Print and shaded views of the part. All mm, measured from the part's lowest x, y and z. A direction names the side the tool comes from. Give positions to 0.01 mm unless a question says otherwise; leave off trailing zeros. Order: outer loops, then holes, each group sorted by start corner. A loop starts at its lowest first (then second) coordinate and runs counter-clockwise, first axis right, second up. Notation, with made-up numbers: (36, 73) - (85, 73) arc R20 ccw to (85, 95) - close; hole circle Ø11 at (48, -12.75). An arc over 180 degrees is marked (long way). Answer in a Markdown table with one row per item.
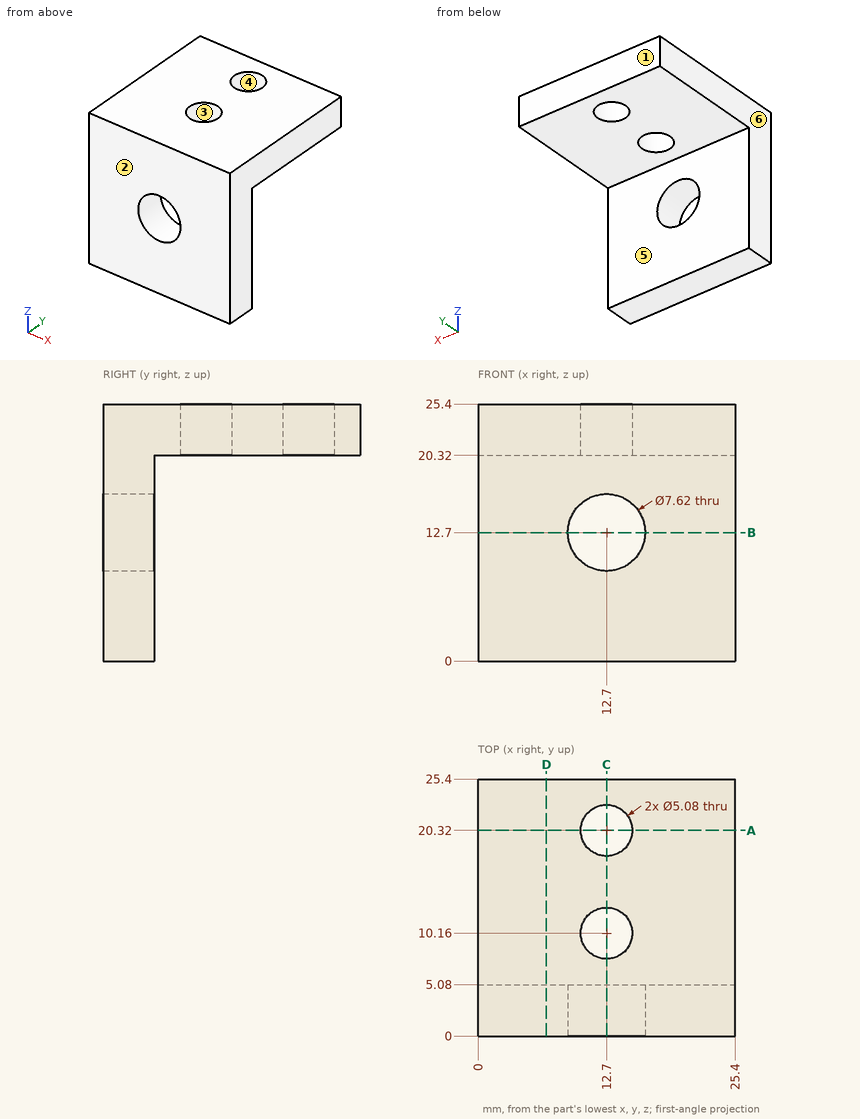
1. Two-plate mould, pull along Y, no slides. Class the marked faces 1, 2, 3 and 4: +Y half, -Y half, draft (parallel to the pull), parting line (faces both ways), or undercut.
Check result:
| item | result |
|---|---|
| face 1 | +Y half |
| face 2 | -Y half |
| face 3 | undercut |
| face 4 | undercut |
2. Probe line 1 (Y direction, x = 12.7, z = 21.7); line 2 (X direction, y = 3.45, z = 12.7); line 3 (Y direction, x = 11.5, z = 22.5). List the from-to ranges inside material, lowest first.
Check result:
| item | result |
|---|---|
| line 1 | y = 0 to 7.62, 12.7 to 17.78, 22.86 to 25.4 |
| line 2 | x = 0 to 8.89, 16.51 to 25.4 |
| line 3 | y = 0 to 7.92, 12.4 to 18.08, 22.56 to 25.4 |
3. Which spindle directions (+Z, -Z, +X, -X, +Y, -Y) get a long thin tool onto all of the face, cutting with end or side? Do the marked faces 5 and 6. Say none if no direction does.
Check result:
| item | result |
|---|---|
| face 5 | -Z, +X, -X, +Y |
| face 6 | +Z, -Z, -X, +Y, -Y |
4. Cut at C-C on x = 12.7. Write the cut outline in (y, z), and give its area (3 significant figures).
Check result:
| item | result |
|---|---|
| outline | (0, 0) - (5.08, 0) - (5.08, 8.89) - (0, 8.89) - close; (0, 16.51) - (5.08, 16.51) - (5.08, 20.32) - (7.62, 20.32) - (7.62, 25.4) - (0, 25.4) - close; (12.7, 20.32) - (17.78, 20.32) - (17.78, 25.4) - (12.7, 25.4) - close; (22.86, 20.32) - (25.4, 20.32) - (25.4, 25.4) - (22.86, 25.4) - close |
| area | 142 mm² |
5. Drop flat-ended pins along their axis: P1, Ø3, axis at x = 9, z = 4.5, coming from the +Y side; P2, Ø6, axis at x = 5.5, y = 23, coming from the -Z side; P3, Ø4.5, axis at x = 12.7, z = 12.7, coming from the -Y side. Give the stop position or say it passes through.
Check result:
| item | result |
|---|---|
| P1 | stops at y = 5.08 |
| P2 | stops at z = 20.32 |
| P3 | passes through |
6. Cut at B-B on z = 12.7. Write the cut outline in (x, y).
Check result:
| item | result |
|---|---|
| outline | (0, 0) - (8.89, 0) - (8.89, 5.08) - (0, 5.08) - close; (16.51, 0) - (25.4, 0) - (25.4, 5.08) - (16.51, 5.08) - close |
7. Cut at A-A on y = 20.32. Write the cut outline in (x, z).
Check result:
| item | result |
|---|---|
| outline | (0, 20.32) - (10.16, 20.32) - (10.16, 25.4) - (0, 25.4) - close; (15.24, 20.32) - (25.4, 20.32) - (25.4, 25.4) - (15.24, 25.4) - close |
8. Cut at D-D on x = 6.75. Write the cut outline in (y, z), and give its area (3 significant figures).
Check result:
| item | result |
|---|---|
| outline | (0, 0) - (5.08, 0) - (5.08, 20.32) - (25.4, 20.32) - (25.4, 25.4) - (0, 25.4) - close |
| area | 232 mm² |
